Part model, mm, in its own coordinate system. A direction names the side the tool comes from. Give positions to 0.01 mm unless a question says otherwise; leave off trailing zeros. Write each loop counter-clockwise with the first axis right and the second up, starting at its lowest first coordinate (ties: lowest second). Pieces come first, ordered by that corner, then holes. Notation, with made-up numbers: (13, 13.5) - (55, 13.5) arc R26 ccw to (55, 35.5) - close; hole circle Ø8 at (25.5, 9). An arc over 180 degrees is marked (long way). Answer in a Markdown table with one row per item. Add a question column.
1. Which spindle directions (+Z, -Z, +X, -X, +Y, -Y) get a long thin tool onto all of the face, cutting with end or side? Do faces 1 (the flat face through (30, 11, 14)), 2 (the flat face through (55, 11, 14)), 3 (the cylindrical face through (62.31, 34.04, 30.28)), 4 (the flat face through (60, 15.318, 30)). Say none if no direction does.
2. Probe line 1 along X through (y, z) = (41, 5); line 2 along Y through (x, z) = (115.5, 2); line 3 along X through (y, z) = (37, 39). List the from-to ranges inside material, lowest first.
3. Band-saw the part on D-D on x = 35. Write the cut outline in (y, z).
4. Band-saw the part on A-A on y = 27. Write the cut outline in (x, z), plus the area to 3 significant figures.
5. Drop flat-ended pins along their axis: pin 1 Ø3 at (x, z) = (36, 31.5) entering from +Y; pin 2 Ø8 at (x, y) = (60.5, 25) entering from +Z; pin 3 Ø3 at (x, z) = (58, 38.5) entering from +Y; pin 4 Ø6 at (x, y) = (20.5, 9) entering from +Z. Give the stop position or say it passes through.
6. Band-saw the part on C-C on y = 35. Write the cut outline in (x, z).
7. Band-saw the part on B-B on z = 42.5. Write the cut outline in (x, y).
```python
from build123d import *

# Parameters (mm, degrees)
BOSS_EXTRUDE1_DEPTH = 50
SKETCH2_W           = 35
SKETCH2_H           = 29.682212161
SKETCH2_R           = 2.5
CUT_EXTRUDE1_DEPTH  = 40


with BuildPart() as part:
    # Sketch1 → Boss-Extrude1 (new body)
    with BuildSketch(Plane.XY):
        Polygon((0, 5), (30, 5), (30, 45), (40, 45), (40, 5), (55, 5), (55, 45), (65, 45), (65, 5), (150, 5), (150, 0), (0, 0), align=None)
    extrude(amount=BOSS_EXTRUDE1_DEPTH)

    # Sketch2 → Cut-Extrude1 (cut)
    with BuildSketch(Plane.XY.offset(50)):
        with Locations((47.5, 30.15889392)):
            Rectangle(SKETCH2_W, SKETCH2_H)
        with Locations((35, 35)):
            Circle(SKETCH2_R, mode=Mode.SUBTRACT)
        with Locations((60, 35)):
            Circle(SKETCH2_R, mode=Mode.SUBTRACT)
    extrude(amount=-CUT_EXTRUDE1_DEPTH, mode=Mode.SUBTRACT)


solid = part.part
```
Values:
| question | item | result |
|---|---|---|
| 1 | face 1 | +Z, -Z, -X, +Y |
| 1 | face 2 | +Z, -Z, +Y |
| 1 | face 3 | +Z |
| 1 | face 4 | +Z, +X, -X |
| 2 | line 1 | x = 30 to 40, 55 to 65 |
| 2 | line 2 | y = 0 to 5 |
| 2 | line 3 | x = 33.5 to 36.5, 58.5 to 61.5 |
| 3 | outline | (0, 0) - (45, 0) - (45, 10) - (37.5, 10) - (37.5, 50) - (32.5, 50) - (32.5, 10) - (15.32, 10) - (15.32, 50) - (0, 50) - close |
| 4 | outline | (30, 0) - (40, 0) - (40, 10) - (30, 10) - close; (55, 0) - (65, 0) - (65, 10) - (55, 10) - close |
| 4 | area | 200 mm² |
| 5 | pin 1 | stops at y = 37.5 |
| 5 | pin 2 | stops at z = 10 |
| 5 | pin 3 | stops at y = 37.45 |
| 5 | pin 4 | passes through |
| 6 | outline | (30, 0) - (40, 0) - (40, 10) - (37.5, 10) - (37.5, 50) - (32.5, 50) - (32.5, 10) - (30, 10) - close; (55, 0) - (65, 0) - (65, 10) - (62.5, 10) - (62.5, 50) - (57.5, 50) - (57.5, 10) - (55, 10) - close |
| 7 | outline | (0, 0) - (150, 0) - (150, 5) - (65, 5) - (65, 15.32) - (55, 15.32) - (55, 5) - (40, 5) - (40, 15.32) - (30, 15.32) - (30, 5) - (0, 5) - close; circle Ø5 at (35, 35); circle Ø5 at (60, 35) |
